Study the drawing (mm; zero at the part's minimum x, y, z) and answer. A direction names the side the tool comes from. Round coordinates to 2 decimals unless told otherwise and drop trailing zeros. Order: outer loops, then holes, each group sorted by start corner. A loop starts at its lowest first (then second) coordinate and runs counter-clockwise, first axis right, second up. Notation, with made-up numbers: (-29.5, 17) -> (27.5, 17) arc R14 cw to (27.5, 38) -> close; hole circle Ø5 at (7, 86). An arc over 180 degrees is marked (long way). Use one line per item in the form item = value.
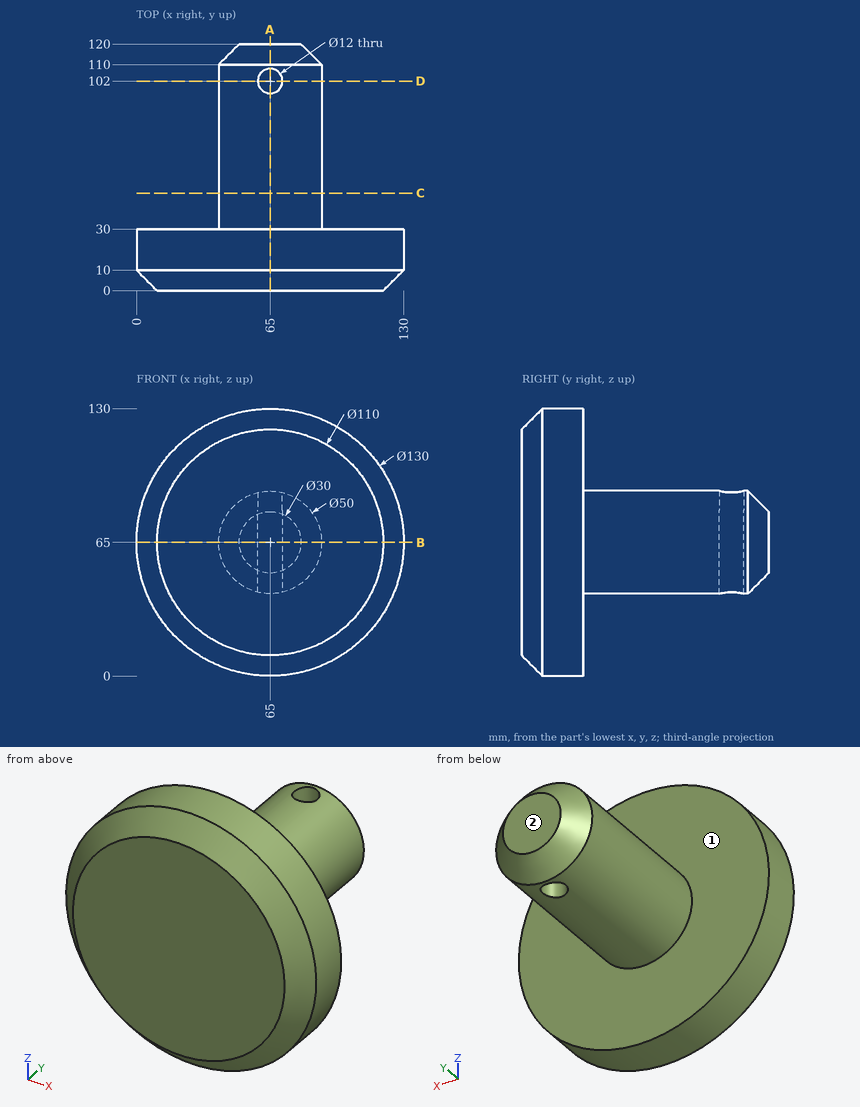
Item 1: The part is cut by section C-C, the plane y = 47.5. Give the vertices of the cut face in (x, z), and give its area (3 significant figures).
Findings:
outline = circle Ø50 at (65, 65)
area = 1,960 mm^2
Item 2: Consider line 1 along Y through (x, z) = (65, 59); line 2 along X through (y, z) = (102, 85); line 3 along Y through (x, z) = (65, 86). Determine where each line is inside the solid, lowest interval first.
Findings:
line_1 = 0 to 96, 108 to 120
line_2 = 50 to 59, 71 to 80
line_3 = 0 to 96, 108 to 114
Item 3: The part is cut by section A-A, the plane x = 65. Give the vertices of the cut face in (y, z), and give its area (3 significant figures).
Findings:
outline = (0, 10) -> (10, 0) -> (30, 0) -> (30, 40) -> (96, 40) -> (96, 90) -> (30, 90) -> (30, 130) -> (10, 130) -> (0, 120) -> close; (108, 40) -> (110, 40) -> (120, 50) -> (120, 80) -> (110, 90) -> (108, 90) -> close
area = 7,600 mm^2
Item 4: Flat-ended cylindrical pins translate along their axes: P1, Ø12, axis at x = 38, z = 36.5, coming from the -Y side; P2, Ø4, axis at x = 37.5, z = 85.5, coming from the +Y side; P3, Ø1, axis at x = 27, y = 12, coming from the -Z side; P4, Ø14, axis at x = 65, y = 102, coming from the +Z side. Find the tip coordinate at first contact, or state that the pin passes through.
Findings:
P1 = 0
P2 = 30
P3 = 11.91
P4 = 90
Item 5: The part is cut by section B-B, the plane z = 65. Give the vertices of the cut face in (x, y), and give its area (3 significant figures).
Findings:
outline = (0, 10) -> (10, 0) -> (120, 0) -> (130, 10) -> (130, 30) -> (90, 30) -> (90, 110) -> (80, 120) -> (50, 120) -> (40, 110) -> (40, 30) -> (0, 30) -> close; hole circle Ø12 at (65, 102)
area = 8,090 mm^2
Item 6: For the marked faces 1 and 2, determine the directions among +Z, -Z, +X, -X, +Y, -Y from which every point of the face is accessible in a straight line to the end or side of a thin tool.
Findings:
face_1 = +Y
face_2 = +Z, -Z, +X, -X, +Y
Item 7: The part is cut by section D-D, the plane y = 102. Give the vertices of the cut face in (x, z), and give its area (3 significant figures).
Findings:
outline = (59, 40.73) -> (59, 89.27) arc R25 ccw to start; (71, 40.73) arc R25 ccw to (71, 89.27) -> close
area = 1,370 mm^2
